```python
from build123d import *

# Parameters (mm, degrees)
SKETCH2_R          = 4
CUT_EXTRUDE1_DEPTH = 12
CUT_EXTRUDE2_REACH = 74
SKETCH3_R          = 4


with BuildPart() as part:
    # Sketch1 → Revolve1 (revolve)
    with BuildSketch(Plane.XY):
        Polygon((-25.700460829, 12), (-25.700460829, 24), (-1.700460829, 24), (-1.700460829, 48), (10.299539171, 48), (10.299539171, 12), align=None)
    revolve(axis=Axis((-11.612903226, 0, 0), (1, 0, 0)))

    # Sketch2 → Cut-Extrude1 (cut)
    with BuildSketch(Plane.ZY.offset(1.700460829)):
        with Locations((0, 36)):
            Circle(SKETCH2_R)
        with Locations((31.176914536, 18)):
            Circle(SKETCH2_R)
        with Locations((31.176914536, -18)):
            Circle(SKETCH2_R)
        with Locations((0, -36)):
            Circle(SKETCH2_R)
        with Locations((-31.176914536, -18)):
            Circle(SKETCH2_R)
        with Locations((-31.176914536, 18)):
            Circle(SKETCH2_R)
    extrude(amount=-CUT_EXTRUDE1_DEPTH, mode=Mode.SUBTRACT)

    # Sketch3 → Cut-Extrude2 (cut, up to next)
    with BuildSketch(Plane.XY.offset(24), mode=Mode.PRIVATE) as cut_extrude2_sk1:
        with Locations((-13.700460829, 0)):
            Circle(SKETCH3_R)
    cut_extrude2_tool1 = extrude(cut_extrude2_sk1.sketch, amount=-CUT_EXTRUDE2_REACH, mode=Mode.PRIVATE) & part.part
    add(cut_extrude2_tool1.solids().sort_by_distance((-13.700461, 0, 24))[0], mode=Mode.SUBTRACT)


solid = part.part
```
Geometry check sheet. Reference: the model listing, model coordinates, mm. A direction names the side the tool comes from. Coordinates: 2 decimals unless noted, no trailing zeros. Write each loop counter-clockwise with the first axis right and the second up, starting at its lowest first coordinate (ties: lowest second). Pieces come first, ordered by that corner, then holes. Notation, with made-up numbers: M -9.75,-4.75 L 49.25,-4.75 A8 cw 49.25,4.25 Z; hole C -7,29 d6. An arc over 180 degrees is marked long. One line per item, written item: value. Start each with the question number.
(1) Sectioned sample at B-B, the plane x = 1. Enter the section's corners in (y, z), and give its area (3 significant figures).
(2) Sectioned sample at C-C, the plane y = 0. Enter the section's corners in (x, z).
(3) Scan lines: line 1 along X through (y, z) = (0, 17.25); line 2 along Y through (x, z) = (4, 1); line 3 along Z through (x, y) = (-12, 0). Record each from-to range of solid material in increasing order. Write a range as [from, to].
(4) Tool access check on faces 1 (the face through (-1.7, 22, -10)), 2 (the face through (-7.952, -2.601, -11.715)). Record the directions out of +Z, -Z, +X, -X, +Y, -Y that give a thin tool (end or side, any length) a straight path to the whole face; none if there is none.
(5) Release check for a two-part mould opening along Z. For faces 3 (the face through (4.216, 39.966, -0.521)), 4 (the face through (-10.005, -1.532, 17.746)), 5 (the face through (4.384, -47.954, 2.11)), 6 (the face through (4.22, -17.82, 27.18)) record: released by +Z, released by -Z, zero draft, split by the parting line, or undercut.
(6) Depth check by flat-ended pin: pin 1 (3 mm diameter, centred on x = -3, y = -9, fed in from -Z); pin 2 (1.5 mm diameter, centred on x = -18, y = -20, fed in from -Z); pin 3 (10 mm diameter, centred on x = 5.5, y = 16, fed in from -Z). Enter the tip coordinate at first touch or a pass-through.
(7) Sectioned sample at D-D, the plane y = 38. Enter the section's corners in (x, z).
(8) Sectioned sample at A-A, the plane z = 0. Enter the section's corners in (x, y), and give its area (3 significant figures).
Filled sheet:
1. outline: C 0,0 d96; hole C -36,0 d8; hole C -18,-31.18 d8; hole C -18,31.18 d8; hole C 0,0 d24; hole C 18,-31.18 d8; hole C 18,31.18 d8; hole C 36,0 d8
1. area: 6,480 mm²
2. outline: M -25.7,-24 L -1.7,-24 L -1.7,-48 L 10.3,-48 L 10.3,-12 L -25.7,-12 Z; M -25.7,12 L -17.7,12 L -17.7,24 L -25.7,24 Z; M -9.7,12 L 10.3,12 L 10.3,48 L -1.7,48 L -1.7,24 L -9.7,24 Z
3. line 1: [-25.7, -17.7], [-9.7, 10.3]
3. line 2: [-47.99, -39.87], [-32.13, -11.96], [11.96, 32.13], [39.87, 47.99]
3. line 3: [-24, -12]
4. face 1: -X
4. face 2: +X, -X
5. face 3: undercut
5. face 4: zero draft
5. face 5: split by the parting line
5. face 6: undercut
6. pin 1: z = -47.29
6. pin 2: z = -14.33
6. pin 3: z = -46.72
7. outline: M -1.7,-29.33 L 10.3,-29.33 L 10.3,-3.46 L -1.7,-3.46 Z; M -1.7,3.46 L 10.3,3.46 L 10.3,29.33 L -1.7,29.33 Z
8. outline: M -25.7,-24 L -1.7,-24 L -1.7,-32 L 10.3,-32 L 10.3,-12 L -25.7,-12 Z; M -25.7,12 L 10.3,12 L 10.3,32 L -1.7,32 L -1.7,24 L -25.7,24 Z; M -1.7,-48 L 10.3,-48 L 10.3,-40 L -1.7,-40 Z; M -1.7,40 L 10.3,40 L 10.3,48 L -1.7,48 Z
8. area: 1,250 mm²
